```python
from build123d import *

# Parameters (mm, degrees)
BOSS_EXTRUDE1_DEPTH = 27.8796339
CUT_EXTRUDE1_DEPTH  = 10
SKETCH3_R           = 7
BOSS_EXTRUDE2_DEPTH = 1


with BuildPart() as part:
    # Sketch1 → Boss-Extrude1 (new body)
    with BuildSketch(Plane.XY):
        with BuildLine():
            Line((3.5, 1.936491673), (3.5, -1.936491673))
            ThreePointArc((3.5, -1.936491673), (-4, 0), (3.5, 1.936491673))
        make_face()
    extrude(amount=-BOSS_EXTRUDE1_DEPTH)

    # Sketch2 → Cut-Extrude1 (cut)
    with BuildSketch(Plane.XY):
        with BuildLine():
            Line((3.5, 1.936491673), (-3.5, 1.936491673))
            ThreePointArc((-3.5, 1.936491673), (0, 4), (3.5, 1.936491673))
        make_face()
        with BuildLine():
            Line((3.5, -1.936491673), (-3.5, -1.936491673))
            ThreePointArc((-3.5, -1.936491673), (0, -4), (3.5, -1.936491673))
        make_face()
    extrude(amount=-CUT_EXTRUDE1_DEPTH, mode=Mode.SUBTRACT)

    # Sketch3 → Boss-Extrude2 (add)
    with BuildSketch(Plane(origin=(0, 0, -27.8796339), x_dir=(-1, 0, 0), z_dir=(0, 0, -1))):
        Circle(SKETCH3_R)
    extrude(amount=BOSS_EXTRUDE2_DEPTH)


solid = part.part
```
CAD build for the part. Positions are in the model's coordinates, mm. A direction names the side the tool comes from. Give positions to 0.01 mm unless a question says otherwise; leave off trailing zeros. Loops run counter-clockwise (first coordinate to the right, second up) from the corner with the lowest first, then second, coordinate; pieces in that order, holes last. Notation, with made-up numbers: (22, 42) -> (41, 42) arc R14 ccw to (41, 62) -> close; hole circle Ø5 at (29.25, -35.5). An arc over 180 degrees is marked (long way). Use a Markdown table: item, result.
1. Flat gauge pins, fed straight in: pin 1 (3 mm diameter, centred on x = 5.5, y = -2, fed in from +Z); pin 2 (3 mm diameter, centred on y = 0, z = -20.5, fed in from +X); pin 3 (2 mm diameter, centred on y = 2, z = -25, fed in from -X); pin 4 (4 mm diameter, centred on x = -3, y = 1, fed in from +Z). Where does each tip first touch, or does it go through?
Check result:
| item | result |
|---|---|
| pin 1 | stops at z = -27.88 |
| pin 2 | stops at x = 3.5 |
| pin 3 | stops at x = -3.87 |
| pin 4 | stops at z = 0 |
2. Slice it at D-D (x = -2.5). List the corners of the cut face in (y, z), plus the area to 3 significant figures.
Check result:
| item | result |
|---|---|
| outline | (-6.54, -28.88) -> (6.54, -28.88) -> (6.54, -27.88) -> (3.12, -27.88) -> (3.12, -10) -> (1.94, -10) -> (1.94, 0) -> (-1.94, 0) -> (-1.94, -10) -> (-3.12, -10) -> (-3.12, -27.88) -> (-6.54, -27.88) -> close |
| area | 163 mm^2 |
3. Which spindle directions (+Z, -Z, +X, -X, +Y, -Y) get a long thin tool onto all of the face, cutting with end or side? Do faces 1 (the cylindrical face through (-6.466, -2.681, -28.373)), 2 (the flat face through (0, -1.936, -5)), 3 (the flat face through (0, 1.936, -5)), 4 (the flat face through (3.5, 0, -14)), 5 (the flat face through (-3, -3, -27.88)). Say none if no direction does.
Check result:
| item | result |
|---|---|
| face 1 | +Z, -Z |
| face 2 | +Z, +X, -X, -Y |
| face 3 | +Z, +X, -X, +Y |
| face 4 | +Z, +X, +Y, -Y |
| face 5 | +Z |
4. Wall check: L1, parallel to Z at x = -1.5, y = -3.75; L2, parallel to Z at x = 0.25, y = -2.75; L3, parallel to X at y = 0.25, z = -9.75. Give the ranges that are in metal, low to high. Write a range as [from, to].
Check result:
| item | result |
|---|---|
| L1 | z = [-28.88, -27.88] |
| L2 | z = [-28.88, -10] |
| L3 | x = [-3.99, 3.5] |
5. Slice it at A-A (x = -0.75). List the corners of the cut face in (y, z).
Check result:
| item | result |
|---|---|
| outline | (-6.96, -28.88) -> (6.96, -28.88) -> (6.96, -27.88) -> (3.93, -27.88) -> (3.93, -10) -> (1.94, -10) -> (1.94, 0) -> (-1.94, 0) -> (-1.94, -10) -> (-3.93, -10) -> (-3.93, -27.88) -> (-6.96, -27.88) -> close |
6. Slice it at C-C (z = -4.5). List the corners of the cut face in (x, y), plus the area to 3 significant figures.
Check result:
| item | result |
|---|---|
| outline | (-3.5, -1.94) -> (3.5, -1.94) -> (3.5, 1.94) -> (-3.5, 1.94) arc R4 ccw to start |
| area | 28.4 mm^2 |
7. Slice it at B-B (y = 0). List the corners of the cut face in (x, z).
Check result:
| item | result |
|---|---|
| outline | (-7, -28.88) -> (7, -28.88) -> (7, -27.88) -> (3.5, -27.88) -> (3.5, 0) -> (-4, 0) -> (-4, -27.88) -> (-7, -27.88) -> close |
